Input: part model. Units: mm. Frame: model coordinates. Round coordinates to 2 decimals unless told otherwise and drop trailing zeros. Write each loop counter-clockwise with the first axis right and the second up, starting at its lowest first coordinate (ties: lowest second). Pieces come first, ordered by that corner, then holes. Notation, with made-up numbers: (13.25, 38) - (21.25, 38) arc R24 cw to (21.25, 64) - close; hole circle Ø11 at (49.5, -14). An arc over 180 degrees is marked (long way). One line per item, written item: value. Start each with the question number.
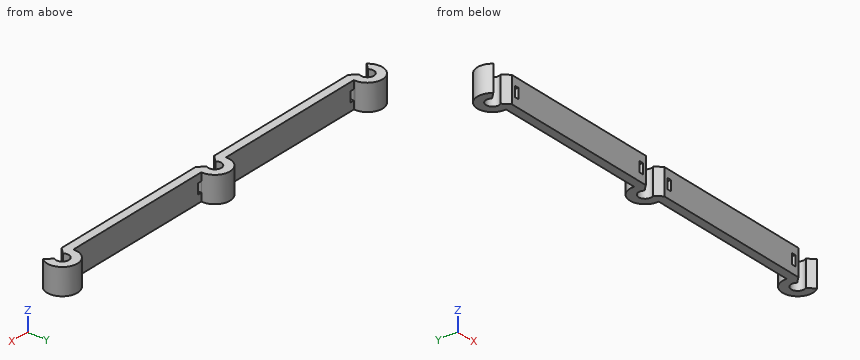
```python
from build123d import *

# Parameters (mm, degrees)
F1_DEPTH = 9
F2_W     = 1.5
F2_H     = 3.5
F3_DEPTH = 3


with BuildPart() as f1:
    # F0 (on Top) → F1 (new body)
    with BuildSketch(Plane.XY):
        with BuildLine():
            ThreePointArc((5.231998, -0.43439), (4.839731, -2.034577), (3.970827, -3.43439))
            Line((3.970827, -3.43439), (61.029173, -3.43439))
            Line((61.029173, -3.43439), (63.163563, -1.3))
            ThreePointArc((63.163563, -1.3), (65, 2.25), (66.836437, -1.3))
            Line((66.836437, -1.3), (68.970827, -3.43439))
            Line((68.970827, -3.43439), (126.029173, -3.43439))
            Line((126.029173, -3.43439), (128.163563, -1.3))
            ThreePointArc((128.163563, -1.3), (130, 2.25), (131.836437, -1.3))
            Line((131.836437, -1.3), (133.970827, -3.43439))
            ThreePointArc((133.970827, -3.43439), (131.627157, 4.991479), (124.768002, -0.43439))
            Line((124.768002, -0.43439), (70.231998, -0.43439))
            ThreePointArc((70.231998, -0.43439), (65, 5.25), (59.768002, -0.43439))
            Line((59.768002, -0.43439), (5.231998, -0.43439))
        make_face()
        with BuildLine():
            ThreePointArc((-1.836437, -1.3), (0, 2.25), (1.836437, -1.3))
            Line((1.836437, -1.3), (3.970827, -3.43439))
            ThreePointArc((3.970827, -3.43439), (4.839731, -2.034577), (5.231998, -0.43439))
            ThreePointArc((5.231998, -0.43439), (5.245498, -0.217381), (5.25, 0))
            ThreePointArc((5.25, 0), (-1.832438, 4.919824), (-3.970827, -3.43439))
            Line((-3.970827, -3.43439), (-1.836437, -1.3))
        make_face()
    extrude(amount=F1_DEPTH)

    # F2 (on face) → F3 (cut, through all)
    with BuildSketch(Plane(origin=(0, -0.43439, 0), x_dir=(-1, 0, 0), z_dir=(0, 1, 0))):
        with Locations((-59.018002, 4.5)):
            Rectangle(F2_W, F2_H)
        with Locations((-70.981998, 4.5)):
            Rectangle(F2_W, F2_H)
        with Locations((-5.981998, 4.5)):
            Rectangle(F2_W, F2_H)
        with Locations((-124.018002, 4.5)):
            Rectangle(F2_W, F2_H)
    extrude(amount=-F3_DEPTH, mode=Mode.SUBTRACT)


solid = f1.part
```
Q1. Cut plane B-B, the plane x = 65. Output: boundary loops of the cut face in (y, z).
Q2. Contact query for flat-ended pins moving along their axis: pin 1 Ø3.5 at (y, z) = (-2, 4.5) entering from +X; pin 2 Ø2.5 at (y, z) = (-1.5, 4.5) entering from -X; pin 3 Ø4.5 at (x, z) = (105.5, 6.5) entering from +Y. Output: stop coordinate, or through.
Q3. Material intervals for probe 1 along X at (y, z) = (0.5, 7.75); probe 2 along X at (y, z) = (-0.5, 0.5); probe 3 along X at (y, z) = (1.75, 1.5), sorted ascending. Write a range as from..to.
Q4. Cut plane A-A, the plane z = 5. Count the separate pieces of the cut face and the enclosed holes in it, and give its area (3 significant figures).
A:
1. outline: (2.25, 0) - (5.25, 0) - (5.25, 9) - (2.25, 9) - close
2. pin 1: stops at x = 135.24
2. pin 2: stops at x = -5.24
2. pin 3: stops at y = -0.43
3. probe 1: x = -5.23..-2.19, 2.19..5.23, 59.77..62.81, 67.19..70.23, 124.77..127.81, 132.19..135.23
3. probe 2: x = -5.23..-2.19, 2.19..62.81, 67.19..127.81, 132.19..135.23
3. probe 3: x = -4.95..-1.41, 1.41..4.95, 60.05..63.59, 66.41..69.95, 125.05..128.59, 131.41..134.95
4. separate pieces: 5
4. enclosed holes: 0
4. area: 467 mm²
